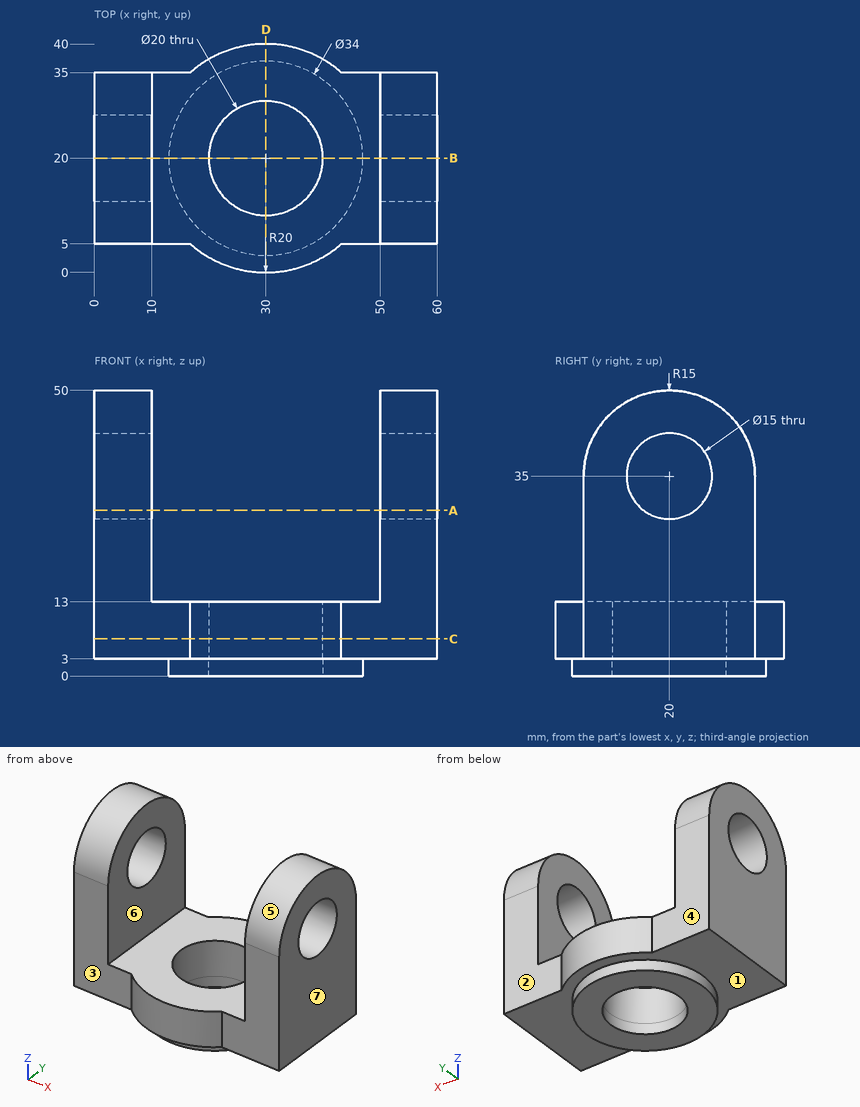
Could you check a few things on this drawing? It's one solid part, dimensions in mm from its lowest x, y, z. A direction names the side the tool comes from. Round coordinates to 2 decimals unless told otherwise and drop trailing zeros. Loops run counter-clockwise (first coordinate to the right, second up) from the corner with the lowest first, then second, coordinate; pieces in that order, holes last.
Q1. I want a section at A-A (z = 29). Write out the boundary of the cut face in (x, y), and give its area (3 significant figures).
Q2. I want a section at C-C (z = 6.5). Write out the boundary of the cut face in (x, y).
Q3. On a 3-axis mill with a long thin cutter (end or side, diameter ignored), from which of +Z, -Z, +X, -X, +Y, -Y can I reach the whole of each face in a straight line? I mean the marked faces 1, 2, 3 and 4. Say none if no direction works.
Q4. For P1, Ø12, axis at x = 23.5, y = 13, coming from the -Z side; P2, Ø2, axis at x = 12.5, y = 34, coming from the -Z side; P3, Ø18.5, axis at x = 54, z = 16.5, coming from the -Y side; P4, Ø4, axis at x = 27, y = 12.5, coming from the +Z side, each with a flat end and sliding along its axis, tell me the tip position at first contact or that it passes through.
Q5. Please list where these lines run through material, in increasing order: L1, parallel to X at y = 9.5, z = 45.5; L2, parallel to Y at x = 30, z = 2; L3, parallel to X at y = 20.5, z = 9.5.
Q6. Thinking about a two-plate mould opening in X: for the marked faces 5, 6 and 7, which applies, pulls with the +X half, pulls with the -X half, needs draft (parallel to the pull), parting line crosses it, or undercut?
Q7. I want a section at D-D (x = 30). Write out the boundary of the cut face in (y, z), and give its area (3 significant figures).
Q8. I want a section at B-B (y = 20). Write out the boundary of the cut face in (x, z), and give its area (3 significant figures).
Answer below:
1. outline: (0, 5) - (10, 5) - (10, 15.5) - (0, 15.5) - close; (0, 24.5) - (10, 24.5) - (10, 35) - (0, 35) - close; (50, 5) - (60, 5) - (60, 15.5) - (50, 15.5) - close; (50, 24.5) - (60, 24.5) - (60, 35) - (50, 35) - close
1. area: 420 mm2
2. outline: (0, 5) - (16.77, 5) arc R20 ccw to (43.23, 5) - (60, 5) - (60, 35) - (43.23, 35) arc R20 ccw to (16.77, 35) - (0, 35) - close; hole circle Ø20 at (30, 20)
3. face 1: -Z
3. face 2: +Z, -Z, +X, +Y
3. face 3: +Z, -Z, -X, -Y
3. face 4: +Z, -Z, -X, +Y
4. P1: stops at z = 0
4. P2: stops at z = 3
4. P3: stops at y = 5
4. P4: stops at z = 13
5. L1: x = 0 to 10, 50 to 60
5. L2: y = 3 to 10, 30 to 37
5. L3: x = 0 to 20.01, 39.99 to 60
6. face 5: needs draft
6. face 6: undercut
6. face 7: pulls with the +X half
7. outline: (0, 3) - (3, 3) - (3, 0) - (10, 0) - (10, 13) - (0, 13) - close; (30, 0) - (37, 0) - (37, 3) - (40, 3) - (40, 13) - (30, 13) - close
7. area: 242 mm2
8. outline: (0, 3) - (13, 3) - (13, 0) - (20, 0) - (20, 13) - (10, 13) - (10, 27.5) - (0, 27.5) - close; (0, 42.5) - (10, 42.5) - (10, 50) - (0, 50) - close; (40, 0) - (47, 0) - (47, 3) - (60, 3) - (60, 27.5) - (50, 27.5) - (50, 13) - (40, 13) - close; (50, 42.5) - (60, 42.5) - (60, 50) - (50, 50) - close
8. area: 882 mm2
